from build123d import *

# Parameters (mm, degrees)
F0_W     = 151
F0_H     = 52
F1_DEPTH = 4
F3_DEPTH = 92
F4_DEPTH = 25


with BuildPart() as f1:
    # F0 (on Top) → F1 (new body)
    with BuildSketch(Plane.XY):
        with Locations((75.5, 26)):
            Rectangle(F0_W, F0_H)
    extrude(amount=F1_DEPTH)

    # F2 (on face) → F3 (join)
    with BuildSketch(Plane.XY.offset(4)):
        Polygon((141, 23), (141, 52), (75.5, 52), (75.5, 0), (151, 0), (151, 23), align=None)
        Polygon((75.5, 0), (75.5, 52), (10, 52), (10, 23), (0, 23), (0, 0), align=None)
    extrude(amount=F3_DEPTH)

    # F2 (on face) → F4 (cut)
    with BuildSketch(Plane.XY.offset(4)):
        with BuildLine():
            Line((6.259378, 40), (0, 40))
            Line((0, 40), (0, 35))
            Line((0, 35), (6.259378, 35))
            ThreePointArc((6.259378, 35), (8.759378, 37.5), (6.259378, 40))
        make_face()
        with BuildLine():
            Line((151, 35), (151, 40))
            Line((151, 40), (144.740622, 40))
            ThreePointArc((144.740622, 40), (142.240622, 37.5), (144.740622, 35))
            Line((144.740622, 35), (151, 35))
        make_face()
    extrude(amount=-F4_DEPTH, mode=Mode.SUBTRACT)


solid = f1.part
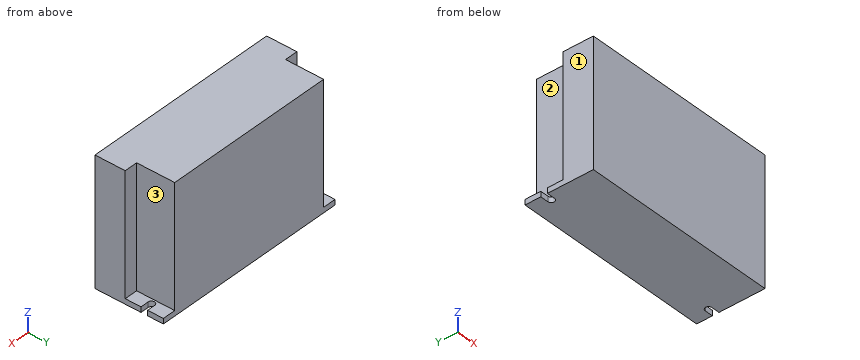
Source: CAD feature listing. Evaluate the final solid. Frame: model axes, mm. Face numbers are marked on the shaded views. A direction names the side the tool comes from. Coordinates: 2 decimals unless noted, no trailing zeros. Loops run counter-clockwise (first coordinate to the right, second up) from the corner with the lowest first, then second, coordinate; pieces in that order, holes last. Notation, with made-up numbers: (22.25, -27) -> (38.25, -27) arc R20 cw to (38.25, 10) -> close; hole circle Ø5 at (36.5, -22.75). An arc over 180 degrees is marked (long way). Answer in a Markdown table with one row per item. Add a question column.
Q1. Reachability of the marked faces 1, 2 and 3 from +Z, -Z, +X, -X, +Y, -Y: full face, straight path, thin tool, end or side. Return the list, or none.
Q2. Section A-A on y = 31. Return the cut outline in (x, z).
Q3. Contact query for flat-ended pins moving along their axis: pin 1 Ø2 at (y, z) = (27.5, 83.5) entering from -X; pin 2 Ø8 at (x, z) = (146.5, 31) entering from +Y; pin 3 Ø5 at (x, y) = (6, 35.5) entering from +Z. Output: stop coordinate, or through.
Q4. Section B-B on z = 61. Return the cut outline in (x, y).
Q5. Ray query, line 1 along X through (y, z) = (44.5, 70.5). Return the intervals inside material, ascending.
Computed values:
| question | item | result |
|---|---|---|
| 1 | face 1 | +Z, -Z, -X, +Y, -Y |
| 1 | face 2 | +Z, -X, +Y |
| 1 | face 3 | +Z, +X, +Y |
| 2 | outline | (0, 0) -> (151, 0) -> (151, 4) -> (141, 4) -> (141, 96) -> (10, 96) -> (10, 4) -> (0, 4) -> close |
| 3 | pin 1 | stops at x = 10 |
| 3 | pin 2 | stops at y = 23 |
| 3 | pin 3 | stops at z = 4 |
| 4 | outline | (0, 0) -> (151, 0) -> (151, 23) -> (141, 23) -> (141, 52) -> (10, 52) -> (10, 23) -> (0, 23) -> close |
| 5 | line 1 | x = 10 to 141 |
